Geometry: final body of the model. Coordinates: model frame, mm. Face numbers are marked on the shaded views. A direction names the side the tool comes from. Give positions to 0.01 mm unless a question says otherwise; leave off trailing zeros. Order: outer loops, then holes, each group sorted by start corner. A loop starts at its lowest first (then second) coordinate and runs counter-clockwise, first axis right, second up. Notation, with made-up numbers: (69.5, 28.5) -> (93.5, 28.5) arc R16 cw to (93.5, 55.5) -> close; hole circle Ø5 at (-25.75, 26.25). An arc over 180 degrees is marked (long way). Write item = value, one per line.
```python
from build123d import *

# Parameters (mm, degrees)
F0_W     = 22.3398831487
F0_H     = 111.7630600929
F1_DEPTH = 1
F2_DEPTH = 1
F3_DEPTH = 1
F4_DEPTH = 14
F5_DEPTH = 14
F6_DEPTH = 1
F7_DEPTH = 1
F8_DEPTH = 5
F9_DEPTH = 5
F11_R    = 0.9999


# Not quite as in the source:
# - a fillet or chamfer is up to 0.001 mm smaller than in the source, because OpenCascade refuses the exact size


with BuildPart() as f1:
    # F0 (on Top) → F1 (new body)
    with BuildSketch(Plane.XY):
        with Locations((-9.3135908246, -6.8099498749)):
            Rectangle(F0_W, F0_H)
    extrude(amount=F1_DEPTH)


with BuildPart() as f2:
    # F2 (new): a face of the model
    f2_faces = [f1.part.faces().sort_by_distance(p)[0] for p in [
        (-9.3135908246, -62.6914799213, 0.5),
    ]]
    extrude(f2_faces, amount=F2_DEPTH)


with BuildPart() as f3:
    # F3 (new): a face of the model
    f3_faces = [f1.part.faces().sort_by_distance(p)[0] for p in [
        (-9.3135908246, 49.0715801716, 0.5),
    ]]
    extrude(f3_faces, amount=F3_DEPTH)


with BuildPart() as f4:
    # F4 (new): a face of the model
    f4_faces = [f3.part.faces().sort_by_distance(p)[0] for p in [
        (-9.3135908246, 49.5715801716, 0),
    ]]
    extrude(f4_faces, amount=F4_DEPTH)


with BuildPart() as f5:
    # F5 (new): a face of the model
    f5_faces = [f2.part.faces().sort_by_distance(p)[0] for p in [
        (-9.3135908246, -63.1914799213, 0),
    ]]
    extrude(f5_faces, amount=F5_DEPTH)


with BuildPart() as f6:
    # F6 (new): a face of the model
    f6_faces = [f5.part.faces().sort_by_distance(p)[0] for p in [
        (-9.3135908246, -63.1914799213, -14),
    ]]
    extrude(f6_faces, amount=F6_DEPTH)


with BuildPart() as f7:
    # F7 (new): a face of the model
    f7_faces = [f4.part.faces().sort_by_distance(p)[0] for p in [
        (-9.3135908246, 49.5715801716, -14),
    ]]
    extrude(f7_faces, amount=F7_DEPTH)


with BuildPart() as f8:
    # F8 (new): a face of the model
    f8_faces = [f6.part.faces().sort_by_distance(p)[0] for p in [
        (-9.3135908246, -62.6914799213, -14.5),
    ]]
    extrude(f8_faces, amount=F8_DEPTH)


with BuildPart() as f9:
    # F9 (new): a face of the model
    f9_faces = [f7.part.faces().sort_by_distance(p)[0] for p in [
        (-9.3135908246, 49.0715801716, -14.5),
    ]]
    extrude(f9_faces, amount=F9_DEPTH)


with BuildPart() as f8_1:
    add(f8.part)

    # F10: union F6, F5, F2, F1, F3, F4, F9, F7
    add(f6.part)
    add(f5.part)
    add(f2.part)
    add(f1.part)
    add(f3.part)
    add(f4.part)
    add(f9.part)
    add(f7.part)

    # F11 (radius 1 in the source; OpenCascade refuses exactly that, so slightly less here)
    f11_edges = [f8_1.edges().sort_by_distance(p)[0] for p in [
        (-9.313591, -62.69148, 0),
        (-20.483532, -63.69148, -7),
        (-9.313591, -63.69148, -15),
        (1.856351, -63.69148, -7),
        (-9.313591, -63.69148, 1),
        (-9.313591, -62.69148, -14),
    ]]
    fillet(f11_edges, radius=F11_R)


solid = f8_1.part
```
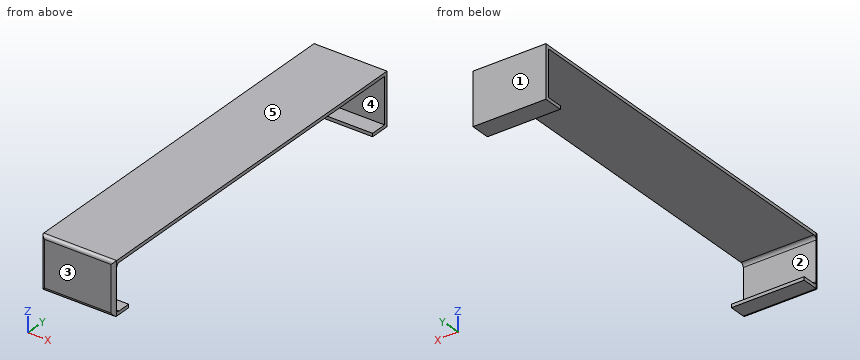
1) First-contact query: P1, Ø3, axis at y = 28.5, z = -2.5, coming from the +X side. Flat tip, straight axial feed; report the tip coordinate or a pass-through.
Check sheet entries:
P1 = through
2) Reachability of the marked faces 1 and 2 from +Z, -Z, +X, -X, +Y, -Y: full face, straight path, thin tool, end or side. Return the list, or none.
Check sheet entries:
face_1 = +Z, -Z, +X, -X, +Y
face_2 = +X, -X
3) Line query: line 1 (Y direction, x = -6.5, z = -5); line 2 (Z direction, x = -8.25, y = 26.5); line 3 (Y direction, x = -17.5, z = -13.75). Output: solid intervals per line, ascending. Write a range as from..to.
Check sheet entries:
line_1 = -63.69..-62.69, 49.07..50.07
line_2 = 0..1
line_3 = -63.69..-62.35, 49.07..50.07
4) Section query C-C (y = -53). Output: boundary loops of the cut face in (x, z), plus the area to 3 significant figures.
Check sheet entries:
outline = (-20.48, 0) -> (1.86, 0) -> (1.86, 1) -> (-20.48, 1) -> close
area = 22.3 mm²
5) Section query B-B (x = -8.75). Output: boundary loops of the cut face in (y, z).
Check sheet entries:
outline = (-63.69, -14) arc R1 ccw to (-62.69, -15) -> (-57.69, -15) -> (-57.69, -14) -> (-61.69, -14) arc R1 cw to (-62.69, -13) -> (-62.69, -1) arc R1 cw to (-61.69, 0) -> (49.07, 0) -> (49.07, -14) -> (44.07, -14) -> (44.07, -15) -> (50.07, -15) -> (50.07, 1) -> (-62.69, 1) arc R1 ccw to (-63.69, 0) -> close
6) Mould query, pull axis Z, two halves, no side actions, for the marked faces 3, 4 and 5. Classes: +Z half, -Z half, draft (parallel to the pull), parting line (faces both ways), or undercut.
Check sheet entries:
face_3 = draft
face_4 = undercut
face_5 = +Z half
